```python
from build123d import *

# Parameters (mm, degrees)
SKETCH2_R           = 1.5
BOSS_EXTRUDE1_DEPTH = 5
BOSS_EXTRUDE2_DEPTH = 35
FILLET1_R           = 2
SKETCH5_W           = 200
SKETCH5_H           = 5
BOSS_EXTRUDE3_DEPTH = 35
FILLET2_R           = 20
FILLET3_R           = 2


with BuildPart() as part:
    # Sketch2 → Boss-Extrude1 (new body)
    # profile 1 of 2: a face of its own
    with BuildSketch(Plane.XY):
        with BuildLine():
            Line((-34.420778608, 16.1), (-49.970391233, 16.1))
            ThreePointArc((-49.970391233, 16.1), (-8.148756355, -51.863742343), (52.5, 0))
            ThreePointArc((52.5, 0), (51.863742343, 8.148756355), (49.970391233, 16.1))
            Line((49.970391233, 16.1), (34.420778608, 16.1))
            ThreePointArc((34.420778608, 16.1), (37.094403804, 8.246526932), (38, 0))
            ThreePointArc((38, 0), (35.577315031, -13.35120426), (28.618176043, -25))
            ThreePointArc((28.618176043, -25), (0, -38), (-28.618176043, -25))
            ThreePointArc((-28.618176043, -25), (-37.626851461, -5.312254619), (-34.420778608, 16.1))
        make_face()
        with Locations((-24.375, -42.218738434)):
            Circle(SKETCH2_R, mode=Mode.SUBTRACT)
        with Locations((-48.75, 0)):
            Circle(SKETCH2_R, mode=Mode.SUBTRACT)
        with Locations((24.375, -42.218738434)):
            Circle(SKETCH2_R, mode=Mode.SUBTRACT)
        with Locations((48.75, 0)):
            Circle(SKETCH2_R, mode=Mode.SUBTRACT)
    # profile 2 of 2: a face of its own
    with BuildSketch(Plane.XY):
        with BuildLine():
            Line((28.618176043, -25), (-28.618176043, -25))
            ThreePointArc((-28.618176043, -25), (0, -38), (28.618176043, -25))
        make_face()
    extrude(amount=BOSS_EXTRUDE1_DEPTH)

    # Sketch4 → Boss-Extrude2 (add)
    with BuildSketch(Plane.XY):
        with BuildLine():
            ThreePointArc((49.970391233, 16.1), (0, -52.5), (-49.970391233, 16.1))
            Line((-49.970391233, 16.1), (-55.2, 16.1))
            ThreePointArc((-55.2, 16.1), (0, -57.5), (55.2, 16.1))
            Line((55.2, 16.1), (49.970391233, 16.1))
        make_face()
    extrude(amount=BOSS_EXTRUDE2_DEPTH)

    # Fillet1
    fillet1_edges = [part.edges().sort_by_distance(p)[0] for p in [
        (34.420778608, 16.1, 2.5),
        (-34.420778608, 16.1, 2.5),
        (-49.970391233, 16.1, 20),
        (-55.2, 16.1, 17.5),
        (55.2, 16.1, 17.5),
        (49.970391233, 16.1, 20),
    ]]
    fillet(fillet1_edges, radius=FILLET1_R)

    # Sketch5 → Boss-Extrude3 (add)
    with BuildSketch(Plane.XY):
        with BuildLine():
            Line((-100, -57.5), (3.75e-07, -57.5))
            ThreePointArc((3.75e-07, -57.5), (-15.165750707, -55.463952307), (-29.257477677, -49.5))
            Line((-29.257477677, -49.5), (-100, -49.5))
            Line((-100, -49.5), (-100, -57.5))
        make_face()
        with BuildLine():
            Line((3.75e-07, -57.5), (100, -57.5))
            Line((100, -57.5), (100, -49.5))
            Line((100, -49.5), (29.257477677, -49.5))
            ThreePointArc((29.257477677, -49.5), (15.165751069, -55.463952208), (3.75e-07, -57.5))
        make_face()
        with Locations((0, -60)):
            Rectangle(SKETCH5_W, SKETCH5_H)
    extrude(amount=BOSS_EXTRUDE3_DEPTH)

    # Fillet2
    fillet2_edges = [part.edges().sort_by_distance(p)[0] for p in [
        (-29.257477677, -49.5, 17.5),
        (29.257477677, -49.5, 17.5),
    ]]
    fillet(fillet2_edges, radius=FILLET2_R)

    # Fillet3
    fillet3_edges = [part.edges().sort_by_distance(p)[0] for p in [
        (100, -49.5, 17.5),
        (-100, -49.5, 17.5),
    ]]
    fillet(fillet3_edges, radius=FILLET3_R)


solid = part.part
```
Model file for the job. Use its own axes, mm. A direction names the side the tool comes from. Round coordinates to 2 decimals unless told otherwise and drop trailing zeros. Write each loop counter-clockwise with the first axis right and the second up, starting at its lowest first coordinate (ties: lowest second). Pieces come first, ordered by that corner, then holes. Notation, with made-up numbers: M -39,41 L 7,41 A7 ccw 7,48 Z; hole C -31.5,11 d4. An arc over 180 degrees is marked long. Put each result on its own line as item: value.
Item 1: Cut at C-C (z = 2). List the corners of the cut face in (x, y) (3 decimals).
Responses:
outline: M -100,-62.5 L 100,-62.5 L 100,-51.5 A2 ccw 98,-49.5 L 71.666,-49.5 A20 cw 53.171,-21.887 A57.5 ccw 55.613,14.608 A2 ccw 53.679,16.1 L 37.432,16.1 A2 ccw 35.561,13.395 A38 cw 28.618,-25 L -28.618,-25 A38 cw -35.561,13.395 A2 ccw -37.432,16.1 L -53.679,16.1 A2 ccw -55.613,14.608 A57.5 ccw -53.171,-21.887 A20 cw -71.666,-49.5 L -98,-49.5 A2 ccw -100,-51.5 Z; hole C -48.75,0 d3; hole C -24.375,-42.219 d3; hole C 24.375,-42.219 d3; hole C 48.75,0 d3
Item 2: Cut at D-D (y = 4.5). List the corners of the cut face in (x, z), and give its area (3 significant figures).
Responses:
outline: M -57.32,0 L -37.73,0 L -37.73,5 L -52.31,5 L -52.31,35 L -57.32,35 Z; M 37.73,0 L 57.32,0 L 57.32,35 L 52.31,35 L 52.31,5 L 37.73,5 Z
area: 497 mm²
Item 3: Tool access for faces 4 (the cylindrical face through (-37.341, -7.044, 2.465)), 5 (the flat face through (85, -49.5, 17)), 6 (the cylindrical face through (1.347, -52.483, 19.79)), 7 (the flat face through (-85, -49.5, 17)), 8 (the flat face through (0, -25, 2)): list every direction of +Z, -Z, +X, -X, +Y, -Y with a clear straight run to the whole face (end or side of a thin tool).
Responses:
face 4: +Z, -Z
face 5: +Z, -Z, +X, +Y
face 6: +Z
face 7: +Z, -Z, -X, +Y
face 8: +Z, -Z, +Y
Item 4: Flat gauge pins, fed straight in: P1, Ø1, axis at y = -27, z = 6.5, coming from the -X side; P2, Ø2.5, axis at x = -24.38, y = -42.22, coming from the -Z side; P3, Ø4, axis at y = -36, z = 30.5, coming from the -X side; P4, Ø2.5, axis at x = 11.5, z = 1.5, coming from the +Y side. Where does each tip first touch, or does it go through?
Responses:
P1: x = -51.89
P2: through
P3: x = -53.56
P4: y = -25
Item 5: Mould opens along X. For faces 1 (the flat face through (-0.7, -25.3, 5)), 2 (the flat face through (-1, -31, 0)), 3 (the cylindrical face through (57.354, -4.099, 17.255)) say: +X half, -X half, draft (parallel to the pull), parting line (faces both ways), or undercut.
Responses:
face 1: undercut
face 2: draft
face 3: +X half
Item 6: Cut at B-B (x = 0). List the corners of the cut face in (y, z), and give its area (4 significant figures).
Responses:
outline: M -62.5,0 L -25,0 L -25,5 L -52.5,5 L -52.5,35 L -62.5,35 Z
area: 487.5 mm²
Item 7: Probe L1, parallel to X at y = -1, z = 4.5; L2, parallel to Y at x = 83.5, z = 3; L3, parallel to Y at x = 0, z = 19.5. List the from-to ranges inside material, lowest first. Write a range as from..to.
Responses:
L1: -57.49..-49.87, -47.63..-37.99, 37.99..47.63, 49.87..57.49
L2: -62.5..-49.5
L3: -62.5..-52.5
Item 8: Cut at A-A (y = -5). List the corners of the cut face in (x, z).
Responses:
outline: M -57.28,0 L -37.67,0 L -37.67,5 L -52.26,5 L -52.26,35 L -57.28,35 Z; M 37.67,0 L 57.28,0 L 57.28,35 L 52.26,35 L 52.26,5 L 37.67,5 Z
